Verification items for the finished model (mm, model axes). A direction names the side the tool comes from. Coordinates: 2 decimals unless noted, no trailing zeros. Write each loop counter-clockwise with the first axis right and the second up, starting at its lowest first coordinate (ties: lowest second). Pieces come first, ordered by that corner, then holes. Notation, with made-up numbers: (-26.5, 22.5) -> (-2.5, 22.5) arc R8 ccw to (-2.5, 35.5) -> close; hole circle Ø7 at (84, 38). An arc over 180 degrees is marked (long way). Answer in a Markdown table with one row per item.
```python
from build123d import *

# Parameters (mm, degrees)
SKETCH1_R           = 20
SKETCH1_R_2         = 3.5
BOSS_EXTRUDE1_DEPTH = 10
FILLET1_R           = 4.5
SKETCH2_R           = 5
CUT_EXTRUDE1_DEPTH  = 2
CUT_EXTRUDE2_START  = -2
SKETCH5_R           = 5
CUT_EXTRUDE2_DEPTH  = 2


with BuildPart() as part:
    # Sketch1 → Boss-Extrude1 (new body)
    with BuildSketch(Plane.XY):
        Circle(SKETCH1_R)
        Circle(SKETCH1_R_2, mode=Mode.SUBTRACT)
    extrude(amount=BOSS_EXTRUDE1_DEPTH)

    # Fillet1
    fillet1_edges = [part.edges().sort_by_distance(p)[0] for p in [
        (-20, 0, 0),
        (-20, 0, 10),
    ]]
    fillet(fillet1_edges, radius=FILLET1_R)

    # Sketch2 → Cut-Extrude1 (cut)
    with BuildSketch(Plane(origin=(0, 0, 0), x_dir=(-1, 0, 0), z_dir=(0, 0, -1))):
        Circle(SKETCH2_R)
    extrude(amount=-CUT_EXTRUDE1_DEPTH, mode=Mode.SUBTRACT)

    # Sketch5 → Cut-Extrude2 (cut)
    with BuildSketch(Plane.XY.offset(10).offset(CUT_EXTRUDE2_START)):
        with Locations(Location((0, 0, 0), (0, 0, 180))):
            Circle(SKETCH5_R)
    extrude(amount=CUT_EXTRUDE2_DEPTH, mode=Mode.SUBTRACT)


solid = part.part
```
1. Sectioned sample at A-A, the plane x = 0. Record the cut outline in (y, z).
Findings below:
| item | result |
|---|---|
| outline | (-20, 4.5) arc R4.5 ccw to (-15.5, 0) -> (-5, 0) -> (-5, 2) -> (-3.5, 2) -> (-3.5, 8) -> (-5, 8) -> (-5, 10) -> (-15.5, 10) arc R4.5 ccw to (-20, 5.5) -> close; (3.5, 2) -> (5, 2) -> (5, 0) -> (15.5, 0) arc R4.5 ccw to (20, 4.5) -> (20, 5.5) arc R4.5 ccw to (15.5, 10) -> (5, 10) -> (5, 8) -> (3.5, 8) -> close |
2. Go/stop test with flat-tipped pins: pin 1 (2 mm diameter, centred on x = 11.5, z = 5.5, fed in from +Y); pin 2 (1.5 mm diameter, centred on y = 4, z = 5, fed in from -X); pin 3 (8 mm diameter, centred on x = 0, y = 0, fed in from +Z). Record where each tip stops, or that it passes through.
Findings below:
| item | result |
|---|---|
| pin 1 | stops at y = 17.02 |
| pin 2 | stops at x = -19.73 |
| pin 3 | stops at z = 8 |
3. Sectioned sample at D-D, the plane z = 3.75. Record the cut outline in (x, y).
Findings below:
| item | result |
|---|---|
| outline | circle Ø39.87 at (0, 0); hole circle Ø7 at (0, 0) |
4. Access from +Z, -Z, +X, -X, +Y, -Y to the whole of each face (thin tool, end or side, straight path). Record for faces 4 (the face through (-3.3, 2.2, 8)), 5 (the face through (-4, 4, 10)), 6 (the face through (-2.2, -3.3, 2)).
Findings below:
| item | result |
|---|---|
| face 4 | +Z |
| face 5 | +Z, +X, -X, +Y, -Y |
| face 6 | -Z |
5. Material ranges on probe 1 along Z at (x, y) = (3, -2); probe 2 along Y at (x, z) = (-3.5, 9.25); probe 3 along X at (y, z) = (1.5, 3.5), recorded low to high. Write a range as from..to.
Findings below:
| item | result |
|---|---|
| probe 1 | z = 2..8 |
| probe 2 | y = -17.64..-3.57, 3.57..17.64 |
| probe 3 | x = -19.83..-3.16, 3.16..19.83 |
6. Sectioned sample at C-C, the plane z = 6.75. Record the cut outline in (x, y), and give its area (3 significant figures).
Findings below:
| item | result |
|---|---|
| outline | circle Ø39.65 at (0, 0); hole circle Ø7 at (0, 0) |
| area | 1,200 mm² |
7. Release check for a two-part mould opening along X. For faces 1 (the face through (-4, 4, 0)), 2 (the face through (-4.336, -19.524, 4.993)), 3 (the face through (5, 0, 9)) record: released by +X, released by -X, zero draft, split by the parting line, or undercut.
Findings below:
| item | result |
|---|---|
| face 1 | zero draft |
| face 2 | split by the parting line |
| face 3 | undercut |
